```python
from build123d import *

# Parameters (mm, degrees)
SKETCH_1_R      = 50
SKETCH_1_R_2    = 37.5
SKETCH_1_R_3    = 3
EXTRUDE_1_DEPTH = 5


with BuildPart() as part:
    # Эскиз1 → Бобышка-Вытянуть1 (new body)
    with BuildSketch(Plane(origin=(0, 0, 0), x_dir=(0, 0, -1), z_dir=(1, 0, 0))):
        Circle(SKETCH_1_R)
        Circle(SKETCH_1_R_2, mode=Mode.SUBTRACT)
        with Locations((0, 43.75)):
            Circle(SKETCH_1_R_3, mode=Mode.SUBTRACT)
        with Locations((13.519493504, 41.608722588)):
            Circle(SKETCH_1_R_3, mode=Mode.SUBTRACT)
        with Locations((25.715604788, 35.394493504)):
            Circle(SKETCH_1_R_3, mode=Mode.SUBTRACT)
        with Locations((35.394493504, 25.715604788)):
            Circle(SKETCH_1_R_3, mode=Mode.SUBTRACT)
        with Locations((41.608722588, 13.519493504)):
            Circle(SKETCH_1_R_3, mode=Mode.SUBTRACT)
        with Locations((43.75, 0)):
            Circle(SKETCH_1_R_3, mode=Mode.SUBTRACT)
        with Locations((41.608722588, -13.519493504)):
            Circle(SKETCH_1_R_3, mode=Mode.SUBTRACT)
        with Locations((35.394493504, -25.715604788)):
            Circle(SKETCH_1_R_3, mode=Mode.SUBTRACT)
        with Locations((25.715604788, -35.394493504)):
            Circle(SKETCH_1_R_3, mode=Mode.SUBTRACT)
        with Locations((13.519493504, -41.608722588)):
            Circle(SKETCH_1_R_3, mode=Mode.SUBTRACT)
        with Locations((0, -43.75)):
            Circle(SKETCH_1_R_3, mode=Mode.SUBTRACT)
        with Locations((-13.519493504, -41.608722588)):
            Circle(SKETCH_1_R_3, mode=Mode.SUBTRACT)
        with Locations((-25.715604788, -35.394493504)):
            Circle(SKETCH_1_R_3, mode=Mode.SUBTRACT)
        with Locations((-35.394493504, -25.715604788)):
            Circle(SKETCH_1_R_3, mode=Mode.SUBTRACT)
        with Locations((-41.608722588, -13.519493504)):
            Circle(SKETCH_1_R_3, mode=Mode.SUBTRACT)
        with Locations((-43.75, 0)):
            Circle(SKETCH_1_R_3, mode=Mode.SUBTRACT)
        with Locations((-41.608722588, 13.519493504)):
            Circle(SKETCH_1_R_3, mode=Mode.SUBTRACT)
        with Locations((-35.394493504, 25.715604788)):
            Circle(SKETCH_1_R_3, mode=Mode.SUBTRACT)
        with Locations((-25.715604788, 35.394493504)):
            Circle(SKETCH_1_R_3, mode=Mode.SUBTRACT)
        with Locations((-13.519493504, 41.608722588)):
            Circle(SKETCH_1_R_3, mode=Mode.SUBTRACT)
    extrude(amount=EXTRUDE_1_DEPTH)


solid = part.part
```
The model under review builds one solid part; all positions refer to its coordinate system, in mm. Round coordinates to 2 decimals unless told otherwise and drop trailing zeros. Loops run counter-clockwise (first coordinate to the right, second up) from the corner with the lowest first, then second, coordinate; pieces in that order, holes last. Notation, with made-up numbers: (34.5, 47.5) - (71.5, 47.5) arc R16 ccw to (71.5, 68.5) - close; hole circle Ø8 at (76, 11). An arc over 180 degrees is marked (long way). Write each question's results on one line, items separated by ' | '. Start each with the question number.
Q1. Wall thickness on line 1 along Z through (x, y) = (4.45, 44); line 2 along Y through (x, z) = (4.55, -13); line 3 along Y through (x, z) = (2.5, -1): over which ranges is each line inside the solid? List them lowest first. Write a range as [from, to].
Q2. Take a section at C-C on x = 3.2. Give the number of separate pieces and of enclosed holes in the cut face, plus the area to 3 significant figures.
Q3. Take a section at A-A on z = 0. Give the boundary of the cut face in (x, y), plus the area to 3 significant figures.
Q4. Draft analysis for pull direction Y (two halves, no side actions). For faces 1 (the cylindrical face through (2.46, 15.02, -47.69)), 2 (the flat face through (5, -37, -11)), 3 (the cylindrical face through (2.46, -33.37, 27.93)), 4 (the cylindrical face through (2.465, -24.814, -38.256)), state which applies: pulls with the +Y half, pulls with the -Y half, needs draft (parallel to the pull), parting line crosses it, or undercut.
Q5. Insertion check: P1, Ø9.5, axis at y = 0, z = 43.75, coming from the +X side; P2, Ø1.5, axis at x = 2, y = -23.5, coming from the -Z side; P3, Ø3, axis at x = 1, z = 26, coming from the +Y side; P4, Ø1.5, axis at x = 1, z = -34.5, coming from the +Y side. Each pin has a flat end and moves straight along its axis. Give the tip position at first contact, or say it passes through.
Data:
1) line 1: z = [-23.75, -15.33], [-11.71, -2.99], [2.99, 11.71], [15.33, 23.75] | line 2: y = [-48.28, -44.56], [-38.65, -35.17], [35.17, 38.65], [44.56, 48.28] | line 3: y = [-49.99, -46.58], [-40.92, -37.49], [37.49, 40.92], [46.58, 49.99]
2) separate pieces: 1 | enclosed holes: 21 | area: 2,870 mm²
3) outline: (0, -50) - (5, -50) - (5, -46.75) - (0, -46.75) - close; (0, -40.75) - (5, -40.75) - (5, -37.5) - (0, -37.5) - close; (0, 37.5) - (5, 37.5) - (5, 40.75) - (0, 40.75) - close; (0, 46.75) - (5, 46.75) - (5, 50) - (0, 50) - close | area: 65.0 mm²
4) face 1: parting line crosses it | face 2: needs draft | face 3: undercut | face 4: undercut
5) P1: stops at x = 5 | P2: stops at z = -44.52 | P3: stops at y = 43.59 | P4: stops at y = 36.89
